from build123d import *

# Parameters (mm, degrees)
BOSS_EXTRUDE1_DEPTH      = 20
CUT_EXTRUDE1_DEPTH       = 17
BOSS_EXTRUDE2_REACH      = 49.969
SKETCH3_R                = 2.5
BOSS_EXTRUDE3_REACH      = 49.969
BOSS_EXTRUDE3_END_RADIUS = 2.5
SKETCH4_R                = 2.5
BOSS_EXTRUDE4_REACH      = 49.969
SKETCH5_R                = 2.5
SKETCH6_R                = 2.2
CUT_EXTRUDE2_DEPTH       = 47.411205543
SKETCH7_R                = 2.2
CUT_EXTRUDE3_DEPTH       = 46.82575695


with BuildPart() as part:
    # Sketch1 → Boss-Extrude1 (new body)
    with BuildSketch(Plane(origin=(0, 0, 0), x_dir=(1, 0, 0), z_dir=(0, 1, 0))):
        Polygon((0, 0), (35, 0), (35, -5), (5, -26), (0, -26), align=None)
    extrude(amount=BOSS_EXTRUDE1_DEPTH)

    # Sketch2 → Cut-Extrude1 (cut)
    with BuildSketch(Plane(origin=(0, 20, 0), x_dir=(1, 0, 0), z_dir=(0, 1, 0))):
        Polygon((35, -3), (3, -3), (3, -26), (5, -26), (35, -5), align=None)
    extrude(amount=-CUT_EXTRUDE1_DEPTH, mode=Mode.SUBTRACT)

    # Sketch3 → Boss-Extrude2 (add, up to next)
    with BuildSketch(Plane.XY.offset(26), mode=Mode.PRIVATE) as boss_extrude2_sk1:
        with Locations((2.5, 2.5)):
            Circle(SKETCH3_R)
    boss_extrude2_tool1 = extrude(boss_extrude2_sk1.sketch, amount=-BOSS_EXTRUDE2_REACH, mode=Mode.PRIVATE) - part.part
    add(boss_extrude2_tool1.solids().sort_by_distance((2.5, 2.5, 26))[0])

    # Boss-Extrude3: up to this cylinder (the profile starts outside it)
    boss_extrude3_end = Plane(origin=(2.5, 2.5, 2.5), z_dir=(0, 0, 1)) * Cylinder(BOSS_EXTRUDE3_END_RADIUS, 105.938, mode=Mode.PRIVATE)
    # Sketch4 → Boss-Extrude3 (add, up to the surface)
    with BuildSketch(Plane(origin=(35, 0, 0), x_dir=(0, 0, -1), z_dir=(1, 0, 0)), mode=Mode.PRIVATE) as boss_extrude3_sk1:
        with Locations((-2.5, 2.5)):
            Circle(SKETCH4_R)
    boss_extrude3_tool1 = extrude(boss_extrude3_sk1.sketch, amount=-BOSS_EXTRUDE3_REACH, mode=Mode.PRIVATE) - boss_extrude3_end
    add(boss_extrude3_tool1.solids().sort_by_distance((35, 2.5, 2.5))[0])

    # Sketch5 → Boss-Extrude4 (add, up to next)
    with BuildSketch(Plane(origin=(0, 20, 0), x_dir=(1, 0, 0), z_dir=(0, 1, 0)), mode=Mode.PRIVATE) as boss_extrude4_sk1:
        with Locations((2.5, -2.5)):
            Circle(SKETCH5_R)
    boss_extrude4_tool1 = extrude(boss_extrude4_sk1.sketch, amount=-BOSS_EXTRUDE4_REACH, mode=Mode.PRIVATE) - part.part
    add(boss_extrude4_tool1.solids().sort_by_distance((2.5, 20, 2.5))[0])

    # Sketch6 → Cut-Extrude2 (cut, through all)
    with BuildSketch(Plane.XY.offset(3)):
        with Locations((10, 10)):
            Circle(SKETCH6_R)
        with Locations((28, 10)):
            Circle(SKETCH6_R)
    extrude(amount=-CUT_EXTRUDE2_DEPTH, mode=Mode.SUBTRACT)

    # Sketch7 → Cut-Extrude3 (cut, through all)
    with BuildSketch(Plane(origin=(3, 0, 0), x_dir=(0, 0, -1), z_dir=(1, 0, 0))):
        with Locations((-13, 10)):
            Circle(SKETCH7_R)
    extrude(amount=-CUT_EXTRUDE3_DEPTH, mode=Mode.SUBTRACT)


solid = part.part
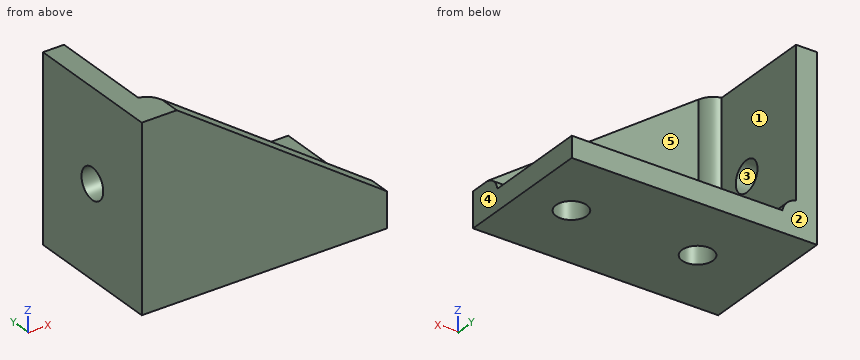
CAD build for the part. Positions are in the model's coordinates, mm. Face numbers are marked on the shaded views. A direction names the side the tool comes from. Coordinates: 2 decimals unless noted, no trailing zeros. Loops run counter-clockwise (first coordinate to the right, second up) from the corner with the lowest first, then second, coordinate; pieces in that order, holes last. Notation, with made-up numbers: (73.25, 56) -> (108.25, 56) arc R21 cw to (108.25, 82) -> close; hole circle Ø11 at (-36.5, 50). An arc over 180 degrees is marked (long way). One line per item, written item: value.
1. Which spindle directions (+Z, -Z, +X, -X, +Y, -Y) get a long thin tool onto all of the face, cutting with end or side? Do the marked faces 4 and 5. Say none if no direction does.
Answers:
face 4: +Z, -Z, +X, +Y, -Y
face 5: +Z, +X, +Y
2. Pull direction Y, two halves, no side cores. Call the marked faces 1, 2 and 3: pulls with the +Y half, pulls with the -Y half, needs draft (parallel to the pull), parting line crosses it, or undercut.
Answers:
face 1: needs draft
face 2: pulls with the +Y half
face 3: undercut
3. Slice it at A-A on x = 10. Write the cut outline in (y, z), and give its area (3 significant figures).
Answers:
outline: (0, 0) -> (7.8, 0) -> (7.8, 3) -> (4.95, 3) arc R2.5 ccw to (3, 4.95) -> (3, 22.5) -> (0, 22.5) -> close; (12.2, 0) -> (20, 0) -> (20, 3) -> (12.2, 3) -> close
area: 108 mm^2
4. Slice it at B-B on y = 10. Write the cut outline in (x, z).
Answers:
outline: (0, 0) -> (7.8, 0) -> (7.8, 3) -> (4.95, 3) arc R2.5 ccw to (3, 4.95) -> (3, 10.8) -> (0, 10.8) -> close; (0, 15.2) -> (3, 15.2) -> (3, 26) -> (0, 26) -> close; (12.2, 0) -> (25.8, 0) -> (25.8, 3) -> (12.2, 3) -> close; (30.2, 0) -> (35, 0) -> (35, 3) -> (30.2, 3) -> close
5. Drill centre lines: line 1 (Y direction, x = 10, z = 1.05); line 2 (Z direction, x = 32, y = 7.75). Where is each one in solid material? Low to high. Write a range as [from, to].
Answers:
line 1: y = [0, 7.8], [12.2, 20]
line 2: z = [0, 3]
6. Slice it at C-C on z = 8.5. Write the cut outline in (x, y), and give its area (3 significant figures).
Answers:
outline: (0, 0) -> (30, 0) -> (30, 3) -> (4.95, 3) arc R2.5 ccw to (3, 4.95) -> (3, 20) -> (0, 20) -> close
area: 144 mm^2
7. Slice it at D-D on z = 13. Write the cut outline in (x, y).
Answers:
outline: (0, 0) -> (23.57, 0) -> (23.57, 3) -> (4.95, 3) arc R2.5 ccw to (3, 4.95) -> (3, 7.8) -> (0, 7.8) -> close; (0, 12.2) -> (3, 12.2) -> (3, 20) -> (0, 20) -> close
8. Flat gauge pins, fed straight in: P1, Ø10, axis at y = 10.5, z = 22, coming from the -X side; P2, Ø4.5, axis at x = 24.5, y = 11, coming from the +Z side; P3, Ø4.5, axis at y = 14, z = 15.5, coming from the +X side; P4, Ø1, axis at y = 14, z = 5, coming from the +X side. Where does each tip first touch, or does it go through?
Answers:
P1: stops at x = 0
P2: stops at z = 3
P3: stops at x = 3
P4: stops at x = 4
